```python
from build123d import *

# Parameters (mm, degrees)
F0_R     = 3.62198
F1_DEPTH = 25
F2_DEPTH = 25


with BuildPart() as f1:
    # F0 (on Front) → F1 (new body)
    with BuildSketch(Plane.XZ):
        Polygon((-24.293795, 32.097615), (-34.310859, 32.097615), (-39.31939, 23.422584), (-34.310859, 14.747553), (-24.293795, 14.747553), (-19.285264, 23.422584), align=None)
        with Locations((-29.302327, 23.422584)):
            Circle(F0_R, mode=Mode.SUBTRACT)
        with Locations((-29.302327, 23.422584)):
            Circle(F0_R)
    extrude(amount=F1_DEPTH)

    # F0 (on Front) → F2 (cut)
    with BuildSketch(Plane.XZ):
        with Locations((-29.302327, 23.422584)):
            Circle(F0_R)
    extrude(amount=F2_DEPTH, mode=Mode.SUBTRACT)


solid = f1.part
```
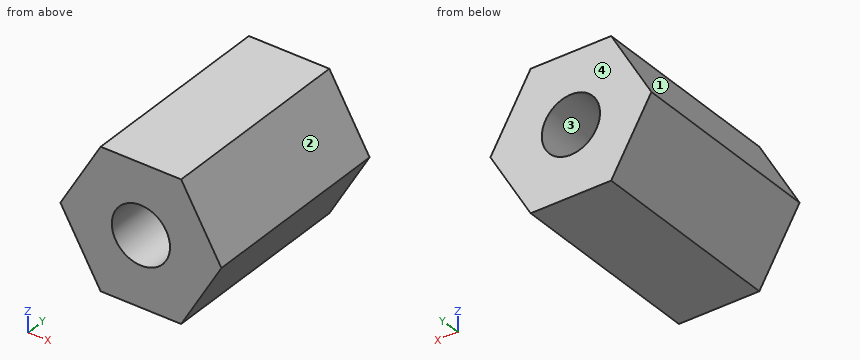
Geometry: final body of the model. Coordinates: model frame, mm. Face numbers are marked on the shaded views. Round coordinates to 2 decimals unless told otherwise and drop trailing zeros. Order: outer loops, then holes, each group sorted by start corner. A loop starts at its lowest first (then second) coordinate and runs counter-clockwise, first axis right, second up. Notation, with made-up numbers: (-24, 11) - (10, 11) arc R30 ccw to (10, 40) - close; hole circle Ø10 at (-30.75, -21). An arc over 180 degrees is marked (long way). Use CSV: the item, a comma, the result in double quotes. Start each with the question number.
Q1. Section query B-B (y = -23). Return loops of the section in (x, z), and give its area (3 significant figures).
Q2. Section query A-A (z = 25.75). Return loops of the section in (x, y).
Q3. Material intervals for line 1 along X through (y, z) = (-3.25, 25.5); line 2 along Z through (x, y) = (-31, -20.75); line 3 along Z through (x, y) = (-30.75, -21.25), sorted ascending. Write a range as from..to.
Q4. Section query D-D (z = 28.5). Return loops of the section in (x, y), and give its area (3 significant figures).
Q5. Section query C-C (x = -30.25). Return loops of the section in (y, z), and give its area (3 significant figures).
Q6. Mould query, pull axis X, two halves, no side actions, for the marked faces 1, 2, 3 and 4. Classes: +X half, -X half, draft (parallel to the pull), parting line (faces both ways), or undercut.
Q7. First-contact query: pin 1 (10 mm diameter, centred on y = -15, z = 29.5, fed in from -X); pin 2 (6 mm diameter, centred on y = -5, z = 27.5, fed in from +X); pin 3 (1.5 mm diameter, centred on x = -23, y = -21, fed in from -Z). Flat tips, straight axial feed; report the tip coordinate or a pass-through.
Result set:
1,outline,"(-39.32, 23.42) - (-34.31, 14.75) - (-24.29, 14.75) - (-19.29, 23.42) - (-24.29, 32.1) - (-34.31, 32.1) - close; hole circle Ø7.24 at (-29.3, 23.42)"
1,area,"219 mm2"
2,outline,"(-37.98, -25) - (-32.08, -25) - (-32.08, 0) - (-37.98, 0) - close; (-26.53, -25) - (-20.63, -25) - (-20.63, 0) - (-26.53, 0) - close"
3,line 1,"x = -38.12..-32.27, -26.34..-20.48"
3,line 2,"z = 14.75..20.22, 26.62..32.1"
3,line 3,"z = 14.75..20.1, 26.74..32.1"
4,outline,"(-36.39, -25) - (-22.22, -25) - (-22.22, 0) - (-36.39, 0) - close"
4,area,"354 mm2"
5,outline,"(-25, 14.75) - (0, 14.75) - (0, 19.93) - (-25, 19.93) - close; (-25, 26.92) - (0, 26.92) - (0, 32.1) - (-25, 32.1) - close"
5,area,"259 mm2"
6,face 1,"-X half"
6,face 2,"+X half"
6,face 3,"undercut"
6,face 4,"draft"
7,pin 1,"stops at x = -38.7"
7,pin 2,"stops at x = -19.91"
7,pin 3,"stops at z = 15.69"
